Source: three-view drawing plus pictorial views. Frame: mm from the lowest corner of the part. Give positions to 0.01 mm unless a question says otherwise; leave off trailing zeros. Write each loop counter-clockwise with the first axis right and the second up, starting at its lowest first coordinate (ties: lowest second). Pieces come first, ordered by that corner, then holes.
Q1. Line query: L1, parallel to Y at x = 11.5, z = 4.5; L2, parallel to Y at x = 9.25, z = 4.25; L3, parallel to X at y = 21, z = 5.75. Output: solid intervals per line, ascending.
Q2. Cut plane B-B on x = 11.5. Return the cut outline in (y, z), plus the area to 3 significant figures.
Q3. Cut plane A-A on y = 25. Return the cut outline in (x, z).
Q4. Cut plane C-C on z = 4.5. Return the cut outline in (x, y), plus the area to 3 significant figures.
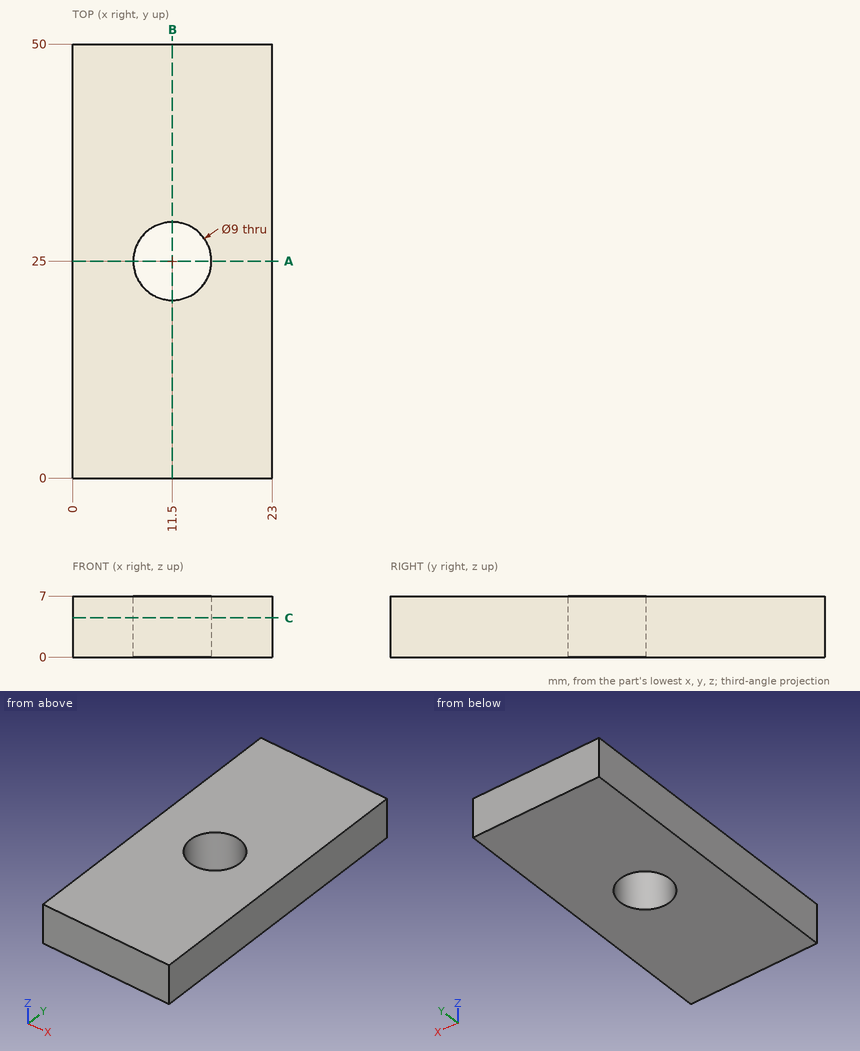
Data:
1. L1: y = 0 to 20.5, 29.5 to 50
1. L2: y = 0 to 21.1, 28.9 to 50
1. L3: x = 0 to 9.44, 13.56 to 23
2. outline: (0, 0) - (20.5, 0) - (20.5, 7) - (0, 7) - close; (29.5, 0) - (50, 0) - (50, 7) - (29.5, 7) - close
2. area: 287 mm2
3. outline: (0, 0) - (7, 0) - (7, 7) - (0, 7) - close; (16, 0) - (23, 0) - (23, 7) - (16, 7) - close
4. outline: (0, 0) - (23, 0) - (23, 50) - (0, 50) - close; hole circle Ø9 at (11.5, 25)
4. area: 1,090 mm2
